Read the model definition and answer for the solid it produces. Units are mm, in the model's axes. Face numbers are marked on the shaded views. A direction names the side the tool comes from. Give positions to 0.01 mm unless a question says otherwise; leave off trailing zeros. Write each loop counter-clockwise with the first axis right and the second up, starting at its lowest first coordinate (ties: lowest second). Pieces come first, ordered by that corner, then holes. Notation, with made-up numbers: (-34.5, 70) -> (-13.5, 70) arc R33 ccw to (-13.5, 101) -> close; hole circle Ø11 at (14.5, -10.5). An arc over 180 degrees is marked (long way). Put each result on its own line as item: value. Start each with the question number.
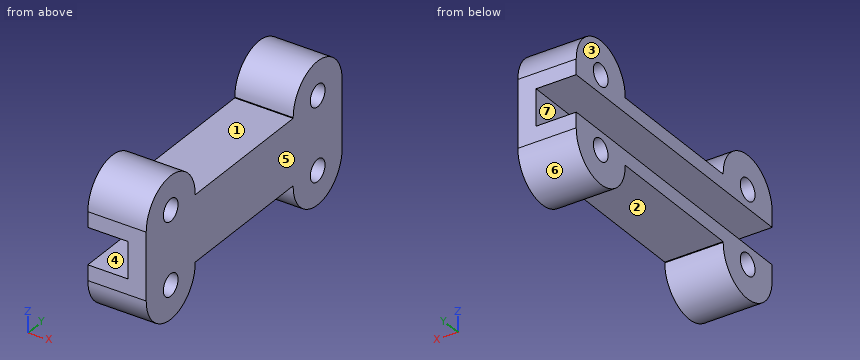
from build123d import *

# Parameters (mm, degrees)
ESQUISSE2_W               = 9
ESQUISSE2_H               = 40
BOSS_EXTRU_1_DEPTH        = 8
ESQUISSE3_W               = 5
ESQUISSE3_H               = 40
ENL_V_MAT_EXTRU_1_DEPTH   = 5.5
ESQUISSE4_W               = 8
ESQUISSE4_H               = 10
BOSS_EXTRU_2_DEPTH        = 0.1
BOSS_EXTRU_5_DEPTH        = 8
ESQUISSE14_R              = 1.5
ENL_V_MAT_EXTRU_4_DEPTH   = 24.583044757
SYM_TRIE5_COPY_1_SKETCH_W = 8
SYM_TRIE5_COPY_1_SKETCH_H = 10
SYM_TRIE5_COPY_1_DEPTH    = 0.1
SYM_TRIE5_COPY_2_DEPTH    = 8
SYM_TRIE5_COPY_3_SKETCH_R = 1.5
SYM_TRIE5_COPY_3_DEPTH    = 24.583044757


with BuildPart() as part:
    # Esquisse2 → Boss.-Extru.1 (new body)
    with BuildSketch(Plane(origin=(0, 0, 0), x_dir=(0, 0, -1), z_dir=(1, 0, 0))):
        Rectangle(ESQUISSE2_W, ESQUISSE2_H)
    extrude(amount=BOSS_EXTRU_1_DEPTH)

    # Esquisse3 → Enlèv. mat.-Extru.1 (cut)
    with BuildSketch(Plane.ZY):
        Rectangle(ESQUISSE3_W, ESQUISSE3_H)
    extrude(amount=-ENL_V_MAT_EXTRU_1_DEPTH, mode=Mode.SUBTRACT)

    # Esquisse4 → Boss.-Extru.2 (add)
    with BuildSketch(Plane(origin=(0, 0, -4.5), x_dir=(-1, 0, 0), z_dir=(0, 0, -1))):
        with Locations((-4, 15)):
            Rectangle(ESQUISSE4_W, ESQUISSE4_H)
    boss_extru_2 = extrude(amount=BOSS_EXTRU_2_DEPTH)

    # Esquisse13 → Boss.-Extru.5 (add)
    with BuildSketch(Plane(origin=(0, 0, 0), x_dir=(0, 0, -1), z_dir=(1, 0, 0))):
        with BuildLine():
            Line((4.6, 10), (4.6, 20))
            ThreePointArc((4.6, 20), (9.6, 15), (4.6, 10))
        make_face()
    boss_extru_5 = extrude(amount=BOSS_EXTRU_5_DEPTH)

    # Esquisse14 → Enlèv. mat.-Extru.4 (cut, through all)
    with BuildSketch(Plane.ZY):
        with Locations((-5, 15)):
            Circle(ESQUISSE14_R)
    enl_v_mat_extru_4 = extrude(amount=-ENL_V_MAT_EXTRU_4_DEPTH, mode=Mode.SUBTRACT)

    # Symétrie4: Boss.-Extru.2, Boss.-Extru.5, Enlèv. mat.-Extru.4 across plane
    add(boss_extru_2.mirror(Plane.XY))
    add(boss_extru_5.mirror(Plane.XY))
    add(enl_v_mat_extru_4.mirror(Plane.XY), mode=Mode.SUBTRACT)

    # Symétrie5: Boss.-Extru.2, Boss.-Extru.5, Enlèv. mat.-Extru.4 across plane
    add(boss_extru_2.mirror(Plane.ZX))
    add(boss_extru_5.mirror(Plane.ZX))
    add(enl_v_mat_extru_4.mirror(Plane.ZX), mode=Mode.SUBTRACT)

    # Symétrie5 copy 1 sketch → Symétrie5 copy 1 (add)
    with BuildSketch(Plane(origin=(0, 0, 4.5), x_dir=(-1, 0, 0), z_dir=(0, 0, 1))):
        with Locations((-4, 15)):
            Rectangle(SYM_TRIE5_COPY_1_SKETCH_W, SYM_TRIE5_COPY_1_SKETCH_H)
    extrude(amount=SYM_TRIE5_COPY_1_DEPTH)

    # Symétrie5 copy 2 sketch → Symétrie5 copy 2 (add)
    with BuildSketch(Plane(origin=(0, 0, 0), x_dir=(0, 0, 1), z_dir=(1, 0, 0))):
        with BuildLine():
            Line((4.6, 10), (4.6, 20))
            ThreePointArc((4.6, 20), (9.6, 15), (4.6, 10))
        make_face()
    extrude(amount=SYM_TRIE5_COPY_2_DEPTH)

    # Symétrie5 copy 3 sketch → Symétrie5 copy 3 (cut, through all)
    with BuildSketch(Plane(origin=(0, 0, 0), x_dir=(0, 0, -1), z_dir=(-1, 0, 0))):
        with Locations((-5, 15)):
            Circle(SYM_TRIE5_COPY_3_SKETCH_R)
    extrude(amount=-SYM_TRIE5_COPY_3_DEPTH, mode=Mode.SUBTRACT)


solid = part.part
1) For a pull along Z with two mould halves and no side action, classify the marked faces 5, 6 and 7 as pulls with the +Z half, pulls with the -Z half, needs draft (parallel to the pull), parting line crosses it, or undercut.
2) A cutting plane is placed at A-A on x = 4. Give the vertices of the cut face in (y, z).
3) Straight lines are drawn through the part: line 1 (Z direction, x = 4.5, y = -15); line 2 (Z direction, x = 6.25, y = -15); line 3 (Y direction, x = 2.25, z = 5). For each, find the intervals that lie inside material, in ascending order. Write a range as [from, to].
4) A cutting plane is placed at C-C on x = 7.5. Give the vertices of the cut face in (y, z).
5) For the marked faces 1, 2, 3 and 4, determine the directions among +Z, -Z, +X, -X, +Y, -Y from which every point of the face is accessible in a straight line to the end or side of a thin tool.
6) Each of these flat-tipped pins is pushed along its axis until it touches: pin 1 Ø3 at (x, y) = (1.5, 9) entering from +Z; pin 2 Ø2.5 at (x, y) = (6, -2) entering from -Z; pin 3 Ø2.5 at (y, z) = (-5.5, -1) entering from -X. Where does it stop, or does it pass through?
7) A cutting plane is placed at B-B on y = -15. Give the vertices of the cut face in (x, z).
8) A cutting plane is placed at D-D on z = -5. Give the vertices of the cut face in (x, y).
Results found:
1. face 5: needs draft
1. face 6: pulls with the -Z half
1. face 7: undercut
2. outline: (-20, -4.6) arc R5 ccw to (-10, -4.6) -> (-10, -4.5) -> (10, -4.5) -> (10, -4.6) arc R5 ccw to (20, -4.6) -> (20, -2.5) -> (-20, -2.5) -> close; (-20, 2.5) -> (20, 2.5) -> (20, 4.6) arc R5 ccw to (10, 4.6) -> (10, 4.5) -> (-10, 4.5) -> (-10, 4.6) arc R5 ccw to (-20, 4.6) -> close; hole circle Ø3 at (-15, -5); hole circle Ø3 at (-15, 5); hole circle Ø3 at (15, -5); hole circle Ø3 at (15, 5)
3. line 1: z = [-9.6, -6.5], [-3.5, -2.5], [2.5, 3.5], [6.5, 9.6]
3. line 2: z = [-9.6, -6.5], [-3.5, 3.5], [6.5, 9.6]
3. line 3: y = [-19.98, -16.5], [-13.5, -10.02], [10.02, 13.5], [16.5, 19.98]
4. outline: (-20, -4.6) arc R5 ccw to (-10, -4.6) -> (-10, -4.5) -> (10, -4.5) -> (10, -4.6) arc R5 ccw to (20, -4.6) -> (20, 4.6) arc R5 ccw to (10, 4.6) -> (10, 4.5) -> (-10, 4.5) -> (-10, 4.6) arc R5 ccw to (-20, 4.6) -> close; hole circle Ø3 at (-15, -5); hole circle Ø3 at (-15, 5); hole circle Ø3 at (15, -5); hole circle Ø3 at (15, 5)
5. face 1: +Z, +X, -X
5. face 2: -Z, +X, -X
5. face 3: +Z, -Z, -X, +Y, -Y
5. face 4: -X, +Y, -Y
6. pin 1: stops at z = 6.78
6. pin 2: stops at z = -4.5
6. pin 3: stops at x = 5.5
7. outline: (0, -9.6) -> (8, -9.6) -> (8, -6.5) -> (0, -6.5) -> close; (0, -3.5) -> (8, -3.5) -> (8, 3.5) -> (0, 3.5) -> (0, 2.5) -> (5.5, 2.5) -> (5.5, -2.5) -> (0, -2.5) -> close; (0, 6.5) -> (8, 6.5) -> (8, 9.6) -> (0, 9.6) -> close
8. outline: (0, -19.98) -> (8, -19.98) -> (8, -16.5) -> (0, -16.5) -> close; (0, -13.5) -> (8, -13.5) -> (8, -10.02) -> (0, -10.02) -> close; (0, 10.02) -> (8, 10.02) -> (8, 13.5) -> (0, 13.5) -> close; (0, 16.5) -> (8, 16.5) -> (8, 19.98) -> (0, 19.98) -> close
